from build123d import *

# Parameters (mm, degrees)
SKETCH1_W           = 35
SKETCH1_H           = 35
SKETCH1_R           = 2
SKETCH1_R_2         = 2.5
BOSS_EXTRUDE1_DEPTH = 10


with BuildPart() as part:
    # Sketch1 → Boss-Extrude1 (new body)
    with BuildSketch(Plane.XY):
        with Locations((2.777777778, 2.470273614)):
            Rectangle(SKETCH1_W, SKETCH1_H)
        with Locations((16.742243872, -11.49419248)):
            Circle(SKETCH1_R, mode=Mode.SUBTRACT)
        with Locations(Location((16.742243872, 16.434739708, 0), (0, 0, 180))):
            Circle(SKETCH1_R, mode=Mode.SUBTRACT)
        with Locations((-11.186688316, 16.434739708)):
            Circle(SKETCH1_R, mode=Mode.SUBTRACT)
        with Locations(Location((-11.186688316, -11.49419248, 0), (0, 0, 180))):
            Circle(SKETCH1_R, mode=Mode.SUBTRACT)
        with Locations(Location((15.277777778, 2.470273614, 0), (0, 0, 180))):
            Circle(SKETCH1_R_2, mode=Mode.SUBTRACT)
        with Locations((-9.722222222, 2.470273614)):
            Circle(SKETCH1_R_2, mode=Mode.SUBTRACT)
    extrude(amount=BOSS_EXTRUDE1_DEPTH)


solid = part.part
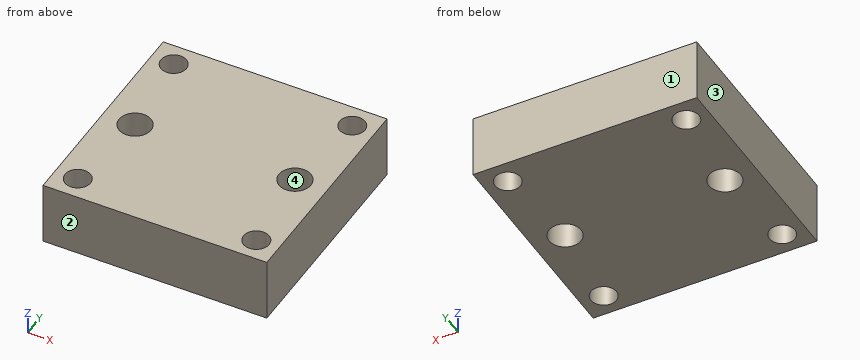
Build history of the part. All positions in model axes, mm. Face numbers are marked on the shaded views. Round coordinates to 2 decimals unless told otherwise and drop trailing zeros. Loops run counter-clockwise (first coordinate to the right, second up) from the corner with the lowest first, then second, coordinate; pieces in that order, holes last. Notation, with made-up numbers: (-34.75, 65.5) -> (10.25, 65.5) arc R15 ccw to (10.25, 76.5) -> close; hole circle Ø8 at (-5, 74.25). An arc over 180 degrees is marked (long way). Use CSV: the item, a comma, the result in double quotes. Start each with the question number.
Q1. Drill centre lines: L1, parallel to Y at x = -12.5, z = 3.5; L2, parallel to X at y = 18, z = 3; L3, parallel to X at y = -12, z = 1.75. Where is each one in solid material? Low to high.
Q2. Mould opens along Y. For the marked faces 1, 2, 3 and 4 say: +Y half, -Y half, draft (parallel to the pull), parting line (faces both ways), or undercut.
Q3. Saw through at D-D on x = 17. Give the cut face in (y, z), and give its area (3 significant figures).
Q4. Saw through at A-A on y = 15. Give the cut face in (x, z), and give its area (3 significant figures).
Q5. Saw through at B-B on x = -11.5. Give the cut face in (y, z), and give its area (3 significant figures).
Q6. Saw through at C-C on z = 8.5. Give the cut face in (x, y), and give its area (3 significant figures).
Q7. Flat gauge pins, fed straight in: pin 1 Ø3 at (x, y) = (-11.19, 16.43) entering from +Z; pin 2 Ø6 at (x, y) = (0.5, 2.5) entering from -Z. Where does each tip first touch, or does it go through?
Solutions:
1,L1,"y = -15.03 to -13, -9.99 to 14.93, 17.94 to 19.97"
1,L2,"x = -14.72 to -12.43, -9.94 to 15.5, 17.99 to 20.28"
1,L3,"x = -14.72 to -13.12, -9.25 to 14.81, 18.68 to 20.28"
2,face 1,"+Y half"
2,face 2,"-Y half"
2,face 3,"draft"
2,face 4,"undercut"
3,outline,"(-15.03, 0) -> (-13.48, 0) -> (-13.48, 10) -> (-15.03, 10) -> close; (-9.51, 0) -> (0.66, 0) -> (0.66, 10) -> (-9.51, 10) -> close; (4.28, 0) -> (14.45, 0) -> (14.45, 10) -> (4.28, 10) -> close; (18.42, 0) -> (19.97, 0) -> (19.97, 10) -> (18.42, 10) -> close"
3,area,"234 mm^2"
4,outline,"(-14.72, 0) -> (-12.58, 0) -> (-12.58, 10) -> (-14.72, 10) -> close; (-9.79, 0) -> (15.35, 0) -> (15.35, 10) -> (-9.79, 10) -> close; (18.14, 0) -> (20.28, 0) -> (20.28, 10) -> (18.14, 10) -> close"
4,area,"294 mm^2"
5,outline,"(-15.03, 0) -> (-13.47, 0) -> (-13.47, 10) -> (-15.03, 10) -> close; (-9.52, 0) -> (0.71, 0) -> (0.71, 10) -> (-9.52, 10) -> close; (4.23, 0) -> (14.46, 0) -> (14.46, 10) -> (4.23, 10) -> close; (18.41, 0) -> (19.97, 0) -> (19.97, 10) -> (18.41, 10) -> close"
5,area,"236 mm^2"
6,outline,"(-14.72, -15.03) -> (20.28, -15.03) -> (20.28, 19.97) -> (-14.72, 19.97) -> close; hole circle Ø4 at (-11.19, -11.49); hole circle Ø4 at (-11.19, 16.43); hole circle Ø5 at (-9.72, 2.47); hole circle Ø5 at (15.28, 2.47); hole circle Ø4 at (16.74, -11.49); hole circle Ø4 at (16.74, 16.43)"
6,area,"1,140 mm^2"
7,pin 1,"passes through"
7,pin 2,"stops at z = 0"
